```python
from build123d import *

# Parameters (mm, degrees)
CYLINDER006_R     = 33
CYLINDER006_DEPTH = 26
CYLINDER005_R     = 35
CYLINDER005_DEPTH = 37
CYLINDER004_R     = 17.2
CYLINDER004_DEPTH = 63
CYLINDER001_R     = 39.5
CYLINDER001_DEPTH = 26
CYLINDER_R        = 43
CYLINDER_DEPTH    = 37
CYLINDER003_R     = 25
CYLINDER003_DEPTH = 49
CHAMFER_SIZE      = 13
CHAMFER001_SIZE   = 3


with BuildPart() as cylinder006:
    # Cylinder006 → Cylinder006 (new body)
    with BuildSketch(Plane.XY.offset(36)):
        Circle(CYLINDER006_R)
    extrude(amount=CYLINDER006_DEPTH)


with BuildPart() as cylinder005:
    # Cylinder005 → Cylinder005 (new body)
    with BuildSketch(Plane.XY):
        Circle(CYLINDER005_R)
    extrude(amount=CYLINDER005_DEPTH)


with BuildPart() as cylinder004:
    # Cylinder004 → Cylinder004 (new body)
    with BuildSketch(Plane.XY.offset(61)):
        Circle(CYLINDER004_R)
    extrude(amount=CYLINDER004_DEPTH)


with BuildPart() as cylinder001:
    # Cylinder001 → Cylinder001 (new body)
    with BuildSketch(Plane.XY.offset(36)):
        Circle(CYLINDER001_R)
    extrude(amount=CYLINDER001_DEPTH)


with BuildPart() as fusion003:
    # Cylinder → Cylinder (new body)
    with BuildSketch(Plane.XY):
        Circle(CYLINDER_R)
    extrude(amount=CYLINDER_DEPTH)

    # Fusion003: union Cylinder001
    add(cylinder001.part)


with BuildPart() as chamfer001:
    # Cylinder003 → Cylinder003 (new body)
    with BuildSketch(Plane.XY.offset(61)):
        Circle(CYLINDER003_R)
    extrude(amount=CYLINDER003_DEPTH)

    # Fusion002: union Fusion003
    add(fusion003.part)


with BuildPart() as chamfer001_1:
    # Fusion002 placement: moved
    add(chamfer001.part.moved(Location((0, 0, 4))))

    # Cut: cut Cylinder004
    add(cylinder004.part, mode=Mode.SUBTRACT)

    # Cut001: cut Cylinder005
    add(cylinder005.part, mode=Mode.SUBTRACT)

    # Cut002: cut Cylinder006
    add(cylinder006.part, mode=Mode.SUBTRACT)

    # Chamfer
    chamfer_edges = [chamfer001_1.edges().sort_by_distance(p)[0] for p in [
        (-25, 0, 66),
    ]]
    chamfer(chamfer_edges, length=CHAMFER_SIZE)

    # Chamfer001
    chamfer001_edges = [chamfer001_1.edges().sort_by_distance(p)[0] for p in [
        (-39.5, 0, 41),
    ]]
    chamfer(chamfer001_edges, length=CHAMFER001_SIZE)


solid = chamfer001_1.part
```
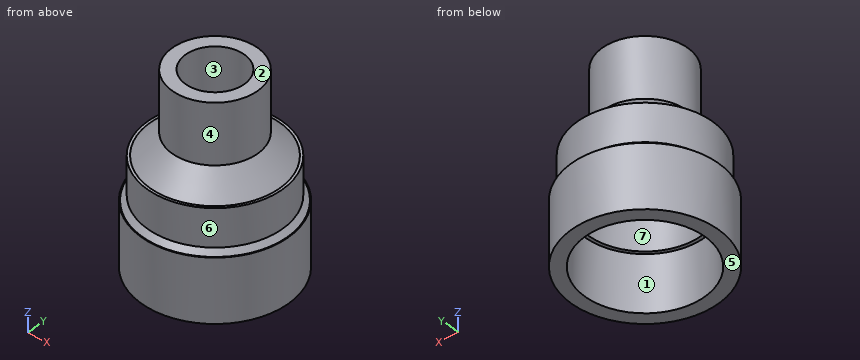
Input: part model. Units: mm. Frame: model coordinates. Face numbers are marked on the shaded views. A direction names the side the tool comes from. Coordinates: 2 decimals unless noted, no trailing zeros. Write each loop counter-clockwise with the first axis right and the second up, starting at its lowest first coordinate (ties: lowest second). Pieces come first, ordered by that corner, then holes. Notation, with made-up numbers: (-10.75, 44.25) - (27.25, 44.25) arc R6 cw to (27.25, 52.25) - close; hole circle Ø11 at (82, -28.75). An arc over 180 degrees is marked (long way). Put each result on its own line as item: value. Start each with the question number.
1) Contact query for flat-ended pins moving along their axis: pin 1 (10 mm diameter, centred on x = -15, z = 81.5, fed in from -Y); pin 2 (1.5 mm diameter, centred on y = -7.5, z = 39.5, fed in from +X); pin 3 (2 mm diameter, centred on x = -11.5, z = 73.5, fed in from -Y). Output: stop coordinate, or through.
2) Mould query, pull axis Y, two halves, no side actions, for the marked faces 1, 2, 3 and 4. Classes: pulls with the +Y half, pulls with the -Y half, needs draft (parallel to the pull), parting line crosses it, or undercut.
3) Cut plane C-C (z = 72.5). Return the cut outline in (x, y).
4) Cut plane A-A (y = 0). Return the cut outline in (x, z), plus the area to 3 significant figures.
5) Ray query, L1, parallel to Y at x = 0, z = 55; L2, parallel to Y at x = -1.5, z = 19. Return the intervals inside material, ascending.
6) Reachability of the marked faces 5, 6 and 7 from +Z, -Z, +X, -X, +Y, -Y: full face, straight path, thin tool, end or side. Return the list, or none.
7) Cut plane D-D (z = 93.5). Return the cut outline in (x, y), plus the area to 3 significant figures.
Resolved:
1. pin 1: stops at y = -23.76
1. pin 2: stops at x = 42.47
1. pin 3: stops at y = -29.39
2. face 1: undercut
2. face 2: needs draft
2. face 3: undercut
2. face 4: parting line crosses it
3. outline: circle Ø63 at (0, 0); hole circle Ø34.4 at (0, 0)
4. outline: (-43, 4) - (-35, 4) - (-35, 37) - (-33, 37) - (-33, 62) - (-17.2, 62) - (-17.2, 114) - (-25, 114) - (-25, 79) - (-38, 66) - (-39.5, 66) - (-39.5, 44) - (-42.5, 41) - (-43, 41) - close; (17.2, 62) - (33, 62) - (33, 37) - (35, 37) - (35, 4) - (43, 4) - (43, 41) - (42.5, 41) - (39.5, 44) - (39.5, 66) - (38, 66) - (25, 79) - (25, 114) - (17.2, 114) - close
4. area: 1,990 mm2
5. L1: y = -39.5 to -33, 33 to 39.5
5. L2: y = -42.97 to -34.97, 34.97 to 42.97
6. face 5: -Z, +X, -X, +Y, -Y
6. face 6: +Z
6. face 7: -Z
7. outline: circle Ø50 at (0, 0); hole circle Ø34.4 at (0, 0)
7. area: 1,030 mm2
